For this review, take the finished solid that the model builds, in its own axes (mm). A direction names the side the tool comes from. Give positions to 0.01 mm unless a question says otherwise; leave off trailing zeros. Loops run counter-clockwise (first coordinate to the right, second up) from the corner with the lowest first, then second, coordinate; pieces in that order, holes last. Notation, with made-up numbers: (65.5, 1.25) -> (81.5, 1.25) arc R9 cw to (81.5, 5.25) -> close; hole circle Ø1 at (83.25, 60). An arc over 180 degrees is marked (long way). Answer as CSV lines item,"result". Start each with the question number.
Item 1: Clearance check with flat-ended pins moving along their axes: P1, Ø1, axis at x = 112.5, z = 61.5, coming from the +Y side; P2, Ø2.5, axis at x = 290.5, z = 47.5, coming from the +Y side; P3, Ø6.5, axis at y = 27.5, z = 49, coming from the +X side. State where each tip first meets the part, or that it passes through.
Item 2: The part is to be moulded in two halves that separate along X. For faces 1 (the face through (110, 15, 46)), 2 (the face through (111.483, 27, 47)), 3 (the face through (248, 15, 0)), say which applies: +X half, -X half, draft (parallel to the pull), parting line (faces both ways), or undercut.
Item 3: Add section B-B on y = 27.5. State the section outline as (x, z) points.
Item 4: Machinability: for faces 4 (the face through (210, 19.942, 47)), 5 (the face through (248, 11, 90)), 6 (the face through (346, 23.901, 47)), which of the approach directions +Z, -Z, +X, -X, +Y, -Y give a long, thin tool a straight path to every point of the face, cutting with its end or side? Answer none if there is none.
Item 5: Add section C-C on x = 130. State the section outline as (y, z) points.
Item 6: For L1, parallel to X at y = 27.5, z = 41; L2, parallel to Z at x = 316, y = 28.75; L3, parallel to Y at x = 340.5, z = 38.5, list the stretches that pass through material, from the lowest coordinate up. Write a range as from..to.
Item 7: Add section A-A on x = 219. State the section outline as (y, z) points.
```python
from build123d import *

# Parameters (mm, degrees)
BOSS_EXTRUDE1_DEPTH = 30
CUT_EXTRUDE1_DEPTH  = 87


with BuildPart() as part:
    # Sketch1 → Boss-Extrude1 (new body)
    with BuildSketch(Plane(origin=(0, 0, 0), x_dir=(1, 0, 0), z_dir=(0, 1, 0))):
        Polygon((250, -90), (110, -90), (110, 0), (390, 0), (390, -90), align=None)
    extrude(amount=BOSS_EXTRUDE1_DEPTH)

    # Sketch3 → Cut-Extrude1 (cut)
    with BuildSketch(Plane.XY.offset(90)):
        Polygon((113.483053539, 23.920467505), (111.483053539, 23.920467505), (111.483053539, 30.115083869), (201.483053539, 30.115083869), (201.483053539, 23.920467505), (199.483053539, 23.920467505), (199.483053539, 19.920467505), (193.9996064, 19.920467505), (193.9996064, 23.920467505), (118.966500679, 23.920467505), (118.966500679, 19.920467505), (113.483053539, 19.920467505), align=None)
        Polygon((302.21010009, 23.900544193), (300.21010009, 23.900544193), (300.21010009, 30.459376692), (390.21010009, 30.459376692), (390.21010009, 23.900544193), (388.21010009, 23.900544193), (388.21010009, 19.900544193), (382.72665295, 19.900544193), (382.72665295, 23.900544193), (307.69354723, 23.900544193), (307.69354723, 19.900544193), (302.21010009, 19.900544193), align=None)
        Polygon((207.348367676, 23.942050812), (205.348367676, 23.942050812), (205.348367676, 30.00297672), (295.348367676, 30.00297672), (295.348367676, 23.942050812), (293.348367676, 23.942050812), (293.348367676, 19.942050812), (287.864920536, 19.942050812), (287.864920536, 23.942050812), (212.831814816, 23.942050812), (212.831814816, 19.942050812), (207.348367676, 19.942050812), align=None)
    extrude(amount=-CUT_EXTRUDE1_DEPTH, mode=Mode.SUBTRACT)


solid = part.part
```
Computed values:
1,P1,"y = 23.92"
1,P2,"y = 19.94"
1,P3,"x = 300.21"
2,face 1,"-X half"
2,face 2,"undercut"
2,face 3,"draft"
3,outline,"(110, 0) -> (390, 0) -> (390, 3) -> (300.21, 3) -> (300.21, 90) -> (295.35, 90) -> (295.35, 3) -> (205.35, 3) -> (205.35, 90) -> (201.48, 90) -> (201.48, 3) -> (111.48, 3) -> (111.48, 90) -> (110, 90) -> close"
4,face 4,"+Z, +Y"
4,face 5,"+Z, +X, -X, +Y, -Y"
4,face 6,"+Z, +X, +Y"
5,outline,"(0, 0) -> (30, 0) -> (30, 3) -> (23.92, 3) -> (23.92, 90) -> (0, 90) -> close"
6,L1,"110..111.48, 201.48..205.35, 295.35..300.21"
6,L2,"0..3"
6,L3,"0..23.9"
7,outline,"(0, 0) -> (30, 0) -> (30, 3) -> (23.94, 3) -> (23.94, 90) -> (0, 90) -> close"
